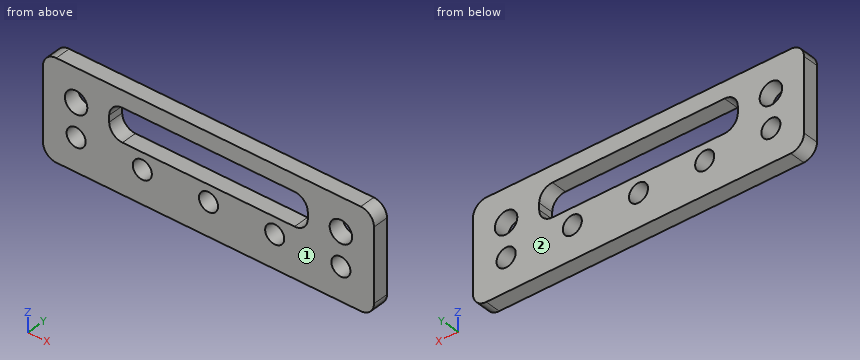
from build123d import *

# Parameters (mm, degrees)
SKETCH1_W             = 63.5
SKETCH1_H             = 19.05
BOSS_EXTRUDE1_DEPTH   = 3
F_6_CLEARANCE_HOLE1_D = 3.6576
F_8_CLEARANCE_HOLE1_D = 4.3053
FILLET1_R             = 2.54
CUT_EXTRUDE1_DEPTH    = 34.283451218


with BuildPart() as part:
    # Sketch1 → Boss-Extrude1 (new body)
    with BuildSketch(Plane(origin=(0, 0, 0), x_dir=(1, 0, 0), z_dir=(0, 1, 0))):
        Rectangle(SKETCH1_W, SKETCH1_H)
    extrude(amount=BOSS_EXTRUDE1_DEPTH)

    # #6 Clearance Hole1 (through all)
    with Locations(Plane(origin=(0, 3, 0), x_dir=(1, 0, 0), z_dir=(0, 1, 0))):
        with Locations((-25.4, 3.175), (0, 3.175), (25.4, 3.175), (12.7, 3.175), (-12.7, 3.175)):
            Hole(F_6_CLEARANCE_HOLE1_D / 2)

    # #8 Clearance Hole1 (through all)
    with Locations(Plane(origin=(0, 3, 0), x_dir=(1, 0, 0), z_dir=(0, 1, 0))):
        with Locations((-25.4, -3.175), (25.4, -3.175)):
            Hole(F_8_CLEARANCE_HOLE1_D / 2)

    # Fillet1
    fillet1_edges = [part.edges().sort_by_distance(p)[0] for p in [
        (-31.75, 1.5, -9.525),
        (31.75, 1.5, -9.525),
        (31.75, 1.5, 9.525),
        (-31.75, 1.5, 9.525),
    ]]
    fillet(fillet1_edges, radius=FILLET1_R)

    # Sketch8 → Cut-Extrude1 (cut, through all)
    with BuildSketch(Plane(origin=(0, 3, 0), x_dir=(1, 0, 0), z_dir=(0, 1, 0))):
        with BuildLine():
            Line((16.51, -6.35), (-16.51, -6.35))
            ThreePointArc((-16.51, -6.35), (-18.306051224, -5.606051224), (-19.05, -3.81))
            Line((-19.05, -3.81), (-19.05, -2.54))
            ThreePointArc((-19.05, -2.54), (-18.306051224, -0.743948776), (-16.51, 0))
            Line((-16.51, 0), (16.51, 0))
            ThreePointArc((16.51, 0), (18.306051224, -0.743948776), (19.05, -2.54))
            Line((19.05, -2.54), (19.05, -3.81))
            ThreePointArc((19.05, -3.81), (18.306051224, -5.606051224), (16.51, -6.35))
        make_face()
    extrude(amount=-CUT_EXTRUDE1_DEPTH, mode=Mode.SUBTRACT)


solid = part.part
Here's how the part is built. I have some questions about the finished solid (model axes, mm). Face numbers are marked on the shaded views. Round coordinates to 2 decimals unless told otherwise and drop trailing zeros. Write each loop counter-clockwise with the first axis right and the second up, starting at its lowest first coordinate (ties: lowest second). Pieces come first, ordered by that corner, then holes.
1. Suppose I cut it at A-A (x = 0). List the corners of the cut face in (y, z) for me (3 decimals), and give its area (3 significant figures).
2. I need wall thicknesses on L1, parallel to Z at x = -12.7, y = 0.9 (3 decimals); L2, parallel to Z at x = 25.4, y = 2.25 (3 decimals); L3, parallel to Z at x = -16, y = 2.1 (3 decimals). Which ranges of each line are inside material? Lowest first, please.
3. Suppose I cut it at D-D (x = 25.4). List the corners of the cut face in (y, z) for me (3 decimals).
4. Suppose I cut it at B-B (y = 0.8). State how many separate pieces and enclosed holes the cut face has, and give its area (3 significant figures).
5. If we mould it in two halves opening along Y, with no side actions, what happens to the marked faces 1 and 2? For each: released by +Y, released by -Y, zero draft, split by the parting line, or undercut.
6. Suppose I cut it at C-C (z = 2). List the corners of the cut face in (x, y) for me, and give its area (3 significant figures).
Answer sheet:
1. outline: (0, -9.525) - (3, -9.525) - (3, -5.004) - (0, -5.004) - close; (0, -1.346) - (3, -1.346) - (3, 0) - (0, 0) - close; (0, 6.35) - (3, 6.35) - (3, 9.525) - (0, 9.525) - close
1. area: 27.1 mm2
2. L1: z = -9.525 to -5.004, -1.346 to 0, 6.35 to 9.525
2. L2: z = -9.525 to -5.004, -1.346 to 1.022, 5.328 to 9.525
2. L3: z = -9.525 to 0, 6.35 to 9.525
3. outline: (0, -9.525) - (3, -9.525) - (3, -5.004) - (0, -5.004) - close; (0, -1.346) - (3, -1.346) - (3, 1.022) - (0, 1.022) - close; (0, 5.328) - (3, 5.328) - (3, 9.525) - (0, 9.525) - close
4. separate pieces: 1
4. enclosed holes: 8
4. area: 886 mm2
5. face 1: released by -Y
5. face 2: released by +Y
6. outline: (-31.75, 0) - (-27.2, 0) - (-27.2, 3) - (-31.75, 3) - close; (-23.6, 0) - (-18.99, 0) - (-18.99, 3) - (-23.6, 3) - close; (18.99, 0) - (23.6, 0) - (23.6, 3) - (18.99, 3) - close; (27.2, 0) - (31.75, 0) - (31.75, 3) - (27.2, 3) - close
6. area: 54.9 mm2
